Geometry: final body of the model. Coordinates: model frame, mm. A direction names the side the tool comes from. Coordinates: 2 decimals unless noted, no trailing zeros. Loops run counter-clockwise (first coordinate to the right, second up) from the corner with the lowest first, then second, coordinate; pieces in that order, holes last. Notation, with made-up numbers: (67, 76.5) - (120, 76.5) arc R8 cw to (120, 80.5) - close; hole circle Ø7 at (51.5, -28). An arc over 180 degrees is marked (long way). Answer in a Markdown table with one row per item.
from build123d import *

# Parameters (mm, degrees)
F0_W      = 140
F0_H      = 30
F1_DEPTH  = 55
F2_W      = 116
F2_H      = 30
F3_DEPTH  = 17.5
F5_D      = 19.6
F7_D      = 6
F9_D      = 6
F10_W     = 56
F10_H     = 30
F10_R     = 3
F11_DEPTH = 24
F12_W     = 56
F12_H     = 30
F12_R     = 3
F13_DEPTH = 24
F15_D     = 5.5
F16_W     = 6
F16_H     = 30.458071
F17_DEPTH = 25


with BuildPart() as f1:
    # F0 (on Top) → F1 (new body)
    with BuildSketch(Plane.XY):
        Rectangle(F0_W, F0_H)
    extrude(amount=F1_DEPTH)

    # F2 (on face) → F3 (cut)
    with BuildSketch(Plane(origin=(0, 0, 0), x_dir=(1, 0, 0), z_dir=(0, 0, -1))):
        Rectangle(F2_W, F2_H)
    extrude(amount=-F3_DEPTH, mode=Mode.SUBTRACT)

    # F5 (through all)
    with Locations(Plane.XZ.offset(15)):
        with Locations((0, 35)):
            Hole(F5_D / 2)

    # F7 (through all)
    with Locations(Plane.XY.offset(55)):
        with Locations((-64, 0)):
            Hole(F7_D / 2)

    # F9 (through all)
    with Locations(Plane.XY.offset(55)):
        with Locations((64, 0)):
            Hole(F9_D / 2)

    # F10 (on face) → F11 (cut)
    with BuildSketch(Plane.XY.offset(55)):
        with Locations((-42, 0)):
            Rectangle(F10_W, F10_H)
        with Locations((-64, 0)):
            Circle(F10_R, mode=Mode.SUBTRACT)
    extrude(amount=-F11_DEPTH, mode=Mode.SUBTRACT)

    # F12 (on face) → F13 (cut)
    with BuildSketch(Plane.XY.offset(55)):
        with Locations((42, 0)):
            Rectangle(F12_W, F12_H)
        with Locations((64, 0)):
            Circle(F12_R, mode=Mode.SUBTRACT)
    extrude(amount=-F13_DEPTH, mode=Mode.SUBTRACT)

    # F15 (through all)
    with Locations(Plane.YZ.offset(14)):
        with Locations((0, 48)):
            Hole(F15_D / 2)

    # F16 (on face) → F17 (cut)
    with BuildSketch(Plane.XY.offset(55)):
        with Locations((0, 0.21546)):
            Rectangle(F16_W, F16_H)
    extrude(amount=-F17_DEPTH, mode=Mode.SUBTRACT)


solid = f1.part
(1) Cut plane A-A on z = 9. Output: boundary loops of the cut face in (x, y), then the cut area to 3 significant figures.
Verdict:
| item | result |
|---|---|
| outline | (-70, -15) - (-58, -15) - (-58, 15) - (-70, 15) - close; (58, -15) - (70, -15) - (70, 15) - (58, 15) - close; hole circle Ø6 at (-64, 0); hole circle Ø6 at (64, 0) |
| area | 663 mm² |
(2) Pull-direction query (X, two-part tool) for faces 5 (the face through (58, 0, 9)), 6 (the face through (-58, 0, 9)), 7 (the face through (-9, 0, 55)), 8 (the face through (14, 0, 43)); classes: pulls with the +X half, pulls with the -X half, needs draft (parallel to the pull), parting line crosses it, or undercut.
Verdict:
| item | result |
|---|---|
| face 5 | undercut |
| face 6 | undercut |
| face 7 | needs draft |
| face 8 | pulls with the +X half |
(3) Cut plane B-B on x = 5. Output: boundary loops of the cut face in (y, z).
Verdict:
| item | result |
|---|---|
| outline | (-15, 17.5) - (15, 17.5) - (15, 26.57) - (-15, 26.57) - close; (-15, 43.43) - (15, 43.43) - (15, 55) - (-15, 55) - close; hole circle Ø5.5 at (0, 48) |
(4) Access query for faces 1 (the face through (42, 0, 31)), 2 (the face through (64, 4, 0)), 3 (the face through (3, 0, 51)), 4 (the face through (-1, 0, 17.5)). Directions: +Z, -Z, +X, -X, +Y, -Y. A direction counts if a zero-diameter tool reaches every point of the face in a straight line with its end or side. Return the directions, or none.
Verdict:
| item | result |
|---|---|
| face 1 | +Z, +X, +Y, -Y |
| face 2 | -Z, +X, -X, +Y, -Y |
| face 3 | +Z, +Y, -Y |
| face 4 | -Z, +Y, -Y |
(5) Cut plane C-C on x = -64. Output: boundary loops of the cut face in (y, z).
Verdict:
| item | result |
|---|---|
| outline | (-15, 0) - (-3, 0) - (-3, 31) - (-15, 31) - close; (3, 0) - (15, 0) - (15, 31) - (3, 31) - close |
(6) Ray query, probe 1 along Z at (x, y) = (-10.5, 0); probe 2 along X at (y, z) = (8.5, 12); probe 3 along X at (y, z) = (-2, 24.5). Return the intervals inside material, ascending.
Verdict:
| item | result |
|---|---|
| probe 1 | z = 17.5 to 45.25, 50.75 to 55 |
| probe 2 | x = -70 to -58, 58 to 70 |
| probe 3 | x = -70 to -66.24, -61.76 to 61.76, 66.24 to 70 |
(7) First-contact query: pin 1 Ø2 at (x, y) = (-31, 10.5) entering from +Z; pin 2 Ø11.5 at (y, z) = (-0.5, 48.5) entering from +X; pin 3 Ø5.5 at (y, z) = (-2, 52.5) entering from -X; pin 4 Ø8 at (x, y) = (64, 0) entering from -Z. Flat tips, straight axial feed; report the tip coordinate or a pass-through.
Verdict:
| item | result |
|---|---|
| pin 1 | stops at z = 31 |
| pin 2 | stops at x = 14 |
| pin 3 | stops at x = -14 |
| pin 4 | stops at z = 0 |
(8) Cut plane D-D on y = 5.75. Output: boundary loops of the cut face in (x, z).
Verdict:
| item | result |
|---|---|
| outline | (-70, 0) - (-58, 0) - (-58, 17.5) - (58, 17.5) - (58, 0) - (70, 0) - (70, 31) - (14, 31) - (14, 55) - (3, 55) - (3, 44.33) arc R9.8 cw (long way) to (-3, 44.33) - (-3, 55) - (-14, 55) - (-14, 31) - (-70, 31) - close |
